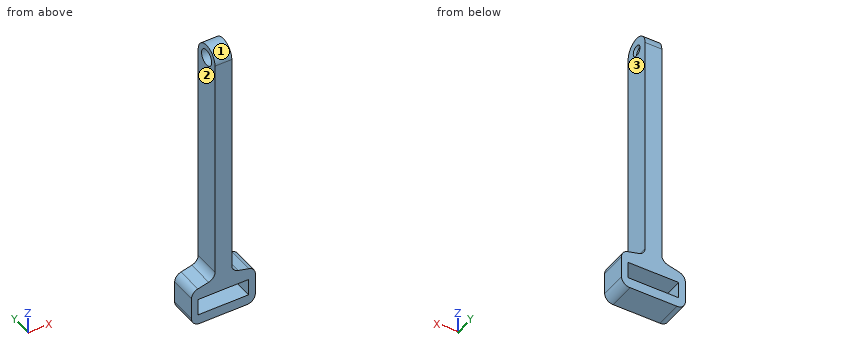
from build123d import *

# Parameters (mm, degrees)
ESQUISSE1_R             = 1.6
BOSS_EXTRU_1_DEPTH      = 5
ESQUISSE3_W             = 15
ESQUISSE3_H             = 5
BOSS_EXTRU_2_DEPTH      = 8
ESQUISSE4_R             = 2.4
ENL_V_MAT_EXTRU_1_DEPTH = 4
CONG_2_R                = 2.5


with BuildPart() as part:
    # Esquisse1 → Boss.-Extru.1 (new body)
    with BuildSketch(Plane(origin=(0, 0, 0), x_dir=(0, 0, -1), z_dir=(1, 0, 0))):
        with BuildLine():
            Line((-30, 4), (41, 4))
            Line((41, 4), (41, -4))
            Line((41, -4), (-30, -4))
            ThreePointArc((-30, -4), (-34, 0), (-30, 4))
        make_face()
        with Locations((-30, 0)):
            Circle(ESQUISSE1_R, mode=Mode.SUBTRACT)
    extrude(amount=BOSS_EXTRU_1_DEPTH)

    # Esquisse3 → Boss.-Extru.2 (add)
    # profile 1 of 3: a face of its own
    with BuildSketch(Plane(origin=(0, 4, 0), x_dir=(1, 0, 0), z_dir=(0, 1, 0))):
        Polygon((5, 41), (12, 41), (12, 52), (-7, 52), (-7, 41), (0, 41), align=None)
        with Locations((2.5, 46.5)):
            Rectangle(ESQUISSE3_W, ESQUISSE3_H, mode=Mode.SUBTRACT)
    # profile 2 of 3: a face of its own
    with BuildSketch(Plane(origin=(0, 4, 0), x_dir=(1, 0, 0), z_dir=(0, 1, 0))):
        Polygon((0, 39.25), (0, 41), (-7, 41), align=None)
    # profile 3 of 3: a face of its own
    with BuildSketch(Plane(origin=(0, 4, 0), x_dir=(1, 0, 0), z_dir=(0, 1, 0))):
        Polygon((12, 41), (5, 41), (5, 39.25), align=None)
    extrude(amount=-BOSS_EXTRU_2_DEPTH)

    # Esquisse4 → Enlèv. mat.-Extru.1 (cut)
    with BuildSketch(Plane.ZY):
        with Locations((30, 0)):
            Circle(ESQUISSE4_R)
    extrude(amount=-ENL_V_MAT_EXTRU_1_DEPTH, mode=Mode.SUBTRACT)

    # Congé2
    cong_2_edges = [part.edges().sort_by_distance(p)[0] for p in [
        (0, 0, -39.25),
        (-7, 0, -41),
        (-7, 0, -52),
        (12, 0, -52),
        (12, 0, -41),
        (5, 0, -39.25),
    ]]
    fillet(cong_2_edges, radius=CONG_2_R)


solid = part.part
Can you work these out from the model? Positions are in its coordinate system, mm. Face numbers are marked on the shaded views. A direction names the side the tool comes from. Round coordinates to 2 decimals unless told otherwise and drop trailing zeros. Write each loop counter-clockwise with the first axis right and the second up, starting at its lowest first coordinate (ties: lowest second). Pieces come first, ordered by that corner, then holes. Notation, with made-up numbers: M 68.25,34.5 L 78.25,34.5 A26 ccw 78.25,73.5 Z; hole C 45,28.5 d2. An arc over 180 degrees is marked long. Use a Markdown table: item, result.
Item 1: I want a section at B-B (x = -2.75). List the corners of the cut face in (y, z) for me.
Found:
| item | result |
|---|---|
| outline | M -4,-52 L 4,-52 L 4,-49 L -4,-49 Z; M -4,-44 L 4,-44 L 4,-39.94 L -4,-39.94 Z |
Item 2: I want a section at C-C (z = -14). List the corners of the cut face in (x, y) for me.
Found:
| item | result |
|---|---|
| outline | M 0,-4 L 5,-4 L 5,4 L 0,4 Z |
Item 3: If I drill on line 1 along Y through (x, z) = (1.65, 30); line 2 along Z through (x, y) = (3.5, 0.5); line 3 along Z through (x, y) = (2, -2), over which ranges is the centre line in solid material (lowest first)? Write a range as [from, to].
Found:
| item | result |
|---|---|
| line 1 | y = [-4, -2.4], [2.4, 4] |
| line 2 | z = [-52, -49], [-44, 27.65], [32.35, 33.97] |
| line 3 | z = [-52, -49], [-44, 28.67], [31.33, 33.46] |
Item 4: I want a section at A-A (y = 0). List the corners of the cut face in (x, z) for me.
Found:
| item | result |
|---|---|
| outline | M -7,-49.5 A2.5 ccw -4.5,-52 L 9.5,-52 A2.5 ccw 12,-49.5 L 12,-42.95 A2.5 ccw 10.11,-40.53 L 6.89,-39.72 A2.5 cw 5,-37.3 L 5,28.4 L 4,28.4 L 4,27.6 L 0,27.6 L 0,-37.3 A2.5 cw -1.89,-39.72 L -5.11,-40.53 A2.5 ccw -7,-42.95 Z; M 0,32.4 L 4,32.4 L 4,31.6 L 5,31.6 L 5,34 L 0,34 Z; hole M -5,-49 L 10,-49 L 10,-44 L -5,-44 Z |
Item 5: Which directions (+Z, -Z, +X, -X, +Y, -Y) give clear straight access to the entire face, cutting with the end or side of a thin tool? Please do the marked faces 1, 2 and 3.
Found:
| item | result |
|---|---|
| face 1 | +Z, +X, -X |
| face 2 | +Z, -X, +Y, -Y |
| face 3 | +Z, +X, +Y, -Y |
Item 6: For pin 1 Ø1.9 at (y, z) = (0, 30) entering from -X; pin 2 Ø1.4 at (y, z) = (1, 30.5) entering from -X; pin 3 Ø3 at (y, z) = (-2.5, -26.5) entering from -X, each with a flat end and sliding along its axis, tell me the tip position at first contact or that it passes through.
Found:
| item | result |
|---|---|
| pin 1 | passes through |
| pin 2 | stops at x = 4 |
| pin 3 | stops at x = 0 |
